Can you work these out from the model? Positions are in its coordinate system, mm. A direction names the side the tool comes from. Round coordinates to 2 decimals unless told otherwise and drop trailing zeros. Order: outer loops, then holes, each group sorted by start corner. A loop starts at its lowest first (then second) coordinate and runs counter-clockwise, first axis right, second up. Notation, with made-up numbers: (-0.75, 89.5) -> (47.25, 89.5) arc R33 cw to (47.25, 117.5) -> close; hole circle Ø7 at (32, 55.25). An arc over 180 degrees is marked (long way). One line per item, written item: value.
```python
from build123d import *

# Parameters (mm, degrees)
F1_DEPTH = 2.54
F2_R     = 5.08
F3_R     = 1.0232120847
F4_DEPTH = 10.16


with BuildPart() as f1:
    # F0 (on Top) → F1 (new body)
    with BuildSketch(Plane.XY):
        Polygon((-25.4, -50.8), (25.4, -50.8), (25.4, -38.1), (12.7, -38.1), (12.7, -17.78), (25.4, -17.78), (25.4, 17.78), (12.7, 17.78), (12.7, 38.1), (25.4, 38.1), (25.4, 50.8), (-25.4, 50.8), (-25.4, 38.1), (-12.7, 38.1), (-12.7, 17.78), (-25.4, 17.78), (-25.4, -17.78), (-12.7, -17.78), (-12.7, -38.1), (-25.4, -38.1), align=None)
    extrude(amount=F1_DEPTH)

    # F2
    f2_edges = [f1.edges().sort_by_distance(p)[0] for p in [
        (25.4, 50.8, 1.27),
        (-25.4, 50.8, 1.27),
        (25.4, -50.8, 1.27),
        (-25.4, -50.8, 1.27),
        (-12.7, -17.78, 1.27),
        (-12.7, -38.1, 1.27),
        (-12.7, 17.78, 1.27),
        (-12.7, 38.1, 1.27),
        (12.7, 38.1, 1.27),
        (12.7, 17.78, 1.27),
        (12.7, -17.78, 1.27),
        (12.7, -38.1, 1.27),
    ]]
    fillet(f2_edges, radius=F2_R)

    # F3 (on Right) → F4 (join, symmetric)
    with BuildSketch(Plane.YZ):
        with BuildLine():
            Line((37.7684151684, 0), (17.5400050426, 0))
            ThreePointArc((17.5400050426, 0), (27.6542101055, -10.1142050629), (37.7684151684, 0))
        make_face()
        with Locations((27.6542101055, -3.3981921151)):
            Circle(F3_R, mode=Mode.SUBTRACT)
        with BuildLine():
            ThreePointArc((-37.7684151684, 0), (-27.6542101055, -10.1142050629), (-17.5400050426, 0))
            Line((-17.5400050426, 0), (-37.7684151684, 0))
        make_face()
        with Locations((-27.6542101055, -3.3981921151)):
            Circle(F3_R, mode=Mode.SUBTRACT)
    extrude(amount=F4_DEPTH, both=True)


solid = f1.part
```
Q1. We'd pull the mould along Y, two halves only. Please class faces 6 (the face through (-0.14, -26.68, -3.09)), 7 (the face through (-10.16, -28, -5)), 8 (the face through (-23.872, -49.351, 1.288)), 9 (the face through (22, -17.78, 1)): released by +Y, released by -Y, zero draft, split by the parting line, or undercut.
Answers below:
face 6: undercut
face 7: zero draft
face 8: released by -Y
face 9: undercut
Q2. I want a section at D-D on y = 8.5. List the corners of the cut face in (x, z) for me.
Answers below:
outline: (-25.4, 0) -> (25.4, 0) -> (25.4, 2.54) -> (-25.4, 2.54) -> close
Q3. Will these pins go through, and if not, where does the flat tip stop? pin 1 Ø2 at (y, z) = (27, 1.5) entering from +X; pin 2 Ø0.8 at (x, z) = (23, 1) entering from -Y; pin 3 Ø6 at (x, z) = (10.5, -8.5) entering from -Y; pin 4 Ø10 at (x, y) = (-5.5, -29.5) entering from -Z.
Answers below:
pin 1: x = 12.7
pin 2: y = -50.26
pin 3: y = -36.13
pin 4: z = -10.11
Q4. I want a section at B-B on x = 15. List the corners of the cut face in (y, z) for me.
Answers below:
outline: (-50.8, 0) -> (-37.27, 0) -> (-37.27, 2.54) -> (-50.8, 2.54) -> close; (-18.61, 0) -> (18.61, 0) -> (18.61, 2.54) -> (-18.61, 2.54) -> close; (37.27, 0) -> (50.8, 0) -> (50.8, 2.54) -> (37.27, 2.54) -> close
Q5. I want a section at C-C on x = -9. List the corners of the cut face in (y, z) for me.
Answers below:
outline: (-50.8, 0) -> (-37.77, 0) arc R10.11 ccw to (-17.54, 0) -> (17.54, 0) arc R10.11 ccw to (37.77, 0) -> (50.8, 0) -> (50.8, 2.54) -> (-50.8, 2.54) -> close; hole circle Ø2.05 at (-27.65, -3.4); hole circle Ø2.05 at (27.65, -3.4)
Q6. On a 3-axis mill with a long thin cutter (end or side, diameter ignored), from which of +Z, -Z, +X, -X, +Y, -Y can I reach the whole of each face in a straight line? I mean faces 1 (the face through (-14.228, 36.651, 1.288)), 2 (the face through (25.4, -42, 1)), 3 (the face through (10.16, -28, -5)), 4 (the face through (14.149, -19.308, 1.288)), 5 (the face through (-10.16, 28, -5)). Say none if no direction works.
Answers below:
face 1: +Z, -Z, -X
face 2: +Z, -Z, +X, +Y, -Y
face 3: -Z, +X, +Y, -Y
face 4: +Z, -Z, +X
face 5: -Z, -X, +Y, -Y
Q7. Please list where these lines run through material, in increasing order: line 1 along Y through (x, z) = (-18, 0.5); line 2 along Y through (x, z) = (-2.5, -0.5); line 3 along Z through (x, y) = (-0.5, 39.5).
Answers below:
line 1: -50.8 to -38.1, -17.78 to 17.78, 38.1 to 50.8
line 2: -37.76 to -17.55, 17.55 to 37.76
line 3: 0 to 2.54
Q8. I want a section at A-A on z = -8.25. List the corners of the cut face in (x, y) for me, plus the area to 3 significant figures.
Answers below:
outline: (-10.16, -33.51) -> (10.16, -33.51) -> (10.16, -21.8) -> (-10.16, -21.8) -> close; (-10.16, 21.8) -> (10.16, 21.8) -> (10.16, 33.51) -> (-10.16, 33.51) -> close
area: 476 mm^2
